Source: CAD feature listing. Evaluate the final solid. Frame: model axes, mm. Face numbers are marked on the shaded views. A direction names the side the tool comes from. Give positions to 0.01 mm unless a question says otherwise; leave off trailing zeros. Loops run counter-clockwise (first coordinate to the right, second up) from the corner with the lowest first, then second, coordinate; pieces in that order, holes last.
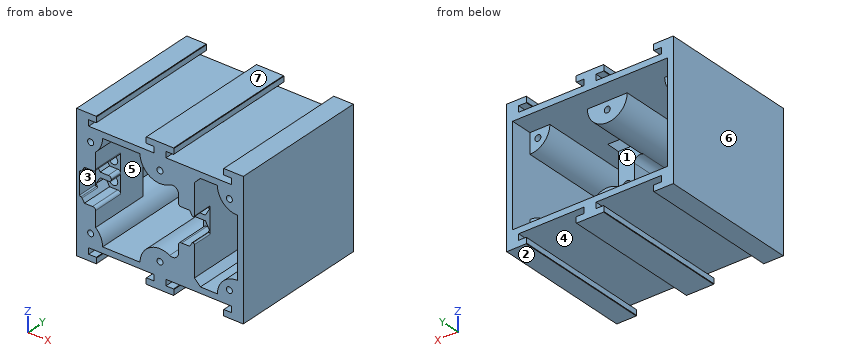
```python
from build123d import *

# Parameters (mm, degrees)
SKETCH1_R             = 1.5
BOSS_EXTRUDE6_DEPTH   = 59
BOSS_EXTRUDE6_2_DEPTH = 59
BOSS_EXTRUDE6_3_DEPTH = 59
BOSS_EXTRUDE6_4_DEPTH = 59
BOSS_EXTRUDE6_5_DEPTH = 59
BOSS_EXTRUDE6_6_DEPTH = 59
SKETCH2_W             = 83.65
SKETCH2_H             = 56
SKETCH2_W_2           = 77.65
SKETCH2_H_2           = 50
BOSS_EXTRUDE7_DEPTH   = 70
SKETCH3_R             = 2.1
SKETCH3_W             = 8
SKETCH3_H             = 50
BOSS_EXTRUDE8_DEPTH   = 30
CHAMFER1_SIZE         = 3
FILLET1_R             = 3
SKETCH4_R             = 2.1
CUT_EXTRUDE2_DEPTH    = 16
FILLET2_R             = 1.3
SKETCH5_W             = 8.8
SKETCH5_H             = 12
CUT_EXTRUDE3_DEPTH    = 10
FILLET3_R             = 0.6
SKETCH6_W             = 6
SKETCH6_H             = 6
BOSS_EXTRUDE9_DEPTH   = 70
CHAMFER3_SIZE         = 0.2


with BuildPart() as part:
    # Sketch1 → Boss-Extrude6 (new body)
    with BuildSketch(Plane(origin=(0, 0, 0), x_dir=(1, 0, 0), z_dir=(0, 1, 0))):
        with BuildLine():
            Line((-38.825, 15), (-38.825, 25))
            Line((-38.825, 25), (-28.825, 25))
            ThreePointArc((-28.825, 25), (-31.753932188, 17.928932188), (-38.825, 15))
        make_face()
        with Locations(Location((-34.825, 21, 0), (0, 0, 270))):
            Circle(SKETCH1_R, mode=Mode.SUBTRACT)
    extrude(amount=BOSS_EXTRUDE6_DEPTH)



with BuildPart() as body_2:
    # Sketch1 → Boss-Extrude6 2 (new body)
    with BuildSketch(Plane(origin=(0, 0, 0), x_dir=(1, 0, 0), z_dir=(0, 1, 0))):
        with BuildLine():
            Line((-38.825, -25), (-28.825, -25))
            ThreePointArc((-28.825, -25), (-31.753932188, -17.928932188), (-38.825, -15))
            Line((-38.825, -15), (-38.825, -25))
        make_face()
        with Locations(Location((-34.825, -21, 0), (0, 0, 270))):
            Circle(SKETCH1_R, mode=Mode.SUBTRACT)
    extrude(amount=BOSS_EXTRUDE6_2_DEPTH)


with BuildPart() as body_3:
    # Sketch1 → Boss-Extrude6 3 (new body)
    with BuildSketch(Plane(origin=(0, 0, 0), x_dir=(1, 0, 0), z_dir=(0, 1, 0))):
        with BuildLine():
            Line((38.825, -25), (38.825, -15))
            ThreePointArc((38.825, -15), (31.753932188, -17.928932188), (28.825, -25))
            Line((28.825, -25), (38.825, -25))
        make_face()
        with Locations(Location((34.825, -21, 0), (0, 0, 270))):
            Circle(SKETCH1_R, mode=Mode.SUBTRACT)
    extrude(amount=BOSS_EXTRUDE6_3_DEPTH)


with BuildPart() as body_4:
    # Sketch1 → Boss-Extrude6 4 (new body)
    with BuildSketch(Plane(origin=(0, 0, 0), x_dir=(1, 0, 0), z_dir=(0, 1, 0))):
        with BuildLine():
            Line((28.825, 25), (38.825, 25))
            Line((38.825, 25), (38.825, 15))
            ThreePointArc((38.825, 15), (31.753932188, 17.928932188), (28.825, 25))
        make_face()
        with Locations(Location((34.825, 21, 0), (0, 0, 270))):
            Circle(SKETCH1_R, mode=Mode.SUBTRACT)
    extrude(amount=BOSS_EXTRUDE6_4_DEPTH)


with BuildPart() as body_5:
    # Sketch1 → Boss-Extrude6 5 (new body)
    with BuildSketch(Plane(origin=(0, 0, 0), x_dir=(1, 0, 0), z_dir=(0, 1, 0))):
        with BuildLine():
            Line((10, -25), (-10, -25))
            ThreePointArc((-10, -25), (0, -15), (10, -25))
        make_face()
        with Locations(Location((0, -21, 0), (0, 0, 270))):
            Circle(SKETCH1_R, mode=Mode.SUBTRACT)
    extrude(amount=BOSS_EXTRUDE6_5_DEPTH)


with BuildPart() as body_6:
    # Sketch1 → Boss-Extrude6 6 (new body)
    with BuildSketch(Plane(origin=(0, 0, 0), x_dir=(1, 0, 0), z_dir=(0, 1, 0))):
        with BuildLine():
            Line((10, 25), (-10, 25))
            ThreePointArc((-10, 25), (0, 15), (10, 25))
        make_face()
        with Locations(Location((0, 21, 0), (0, 0, 270))):
            Circle(SKETCH1_R, mode=Mode.SUBTRACT)
    extrude(amount=BOSS_EXTRUDE6_6_DEPTH)


with BuildPart() as part_1:
    add(part.part)

    add(body_2.part)  # Boss-Extrude7 merges body 2

    add(body_3.part)  # Boss-Extrude7 merges body 3

    add(body_4.part)  # Boss-Extrude7 merges body 4

    add(body_5.part)  # Boss-Extrude7 merges body 5

    add(body_6.part)  # Boss-Extrude7 merges body 6
    # Sketch2 → Boss-Extrude7 (add)
    with BuildSketch(Plane(origin=(0, 0, 0), x_dir=(1, 0, 0), z_dir=(0, 1, 0))):
        Rectangle(SKETCH2_W, SKETCH2_H)
        Rectangle(SKETCH2_W_2, SKETCH2_H_2, mode=Mode.SUBTRACT)
    extrude(amount=BOSS_EXTRUDE7_DEPTH)

    # Sketch3 → Boss-Extrude8 (add)
    # profile 1 of 2: a face of its own
    with BuildSketch(Plane(origin=(0, 0, 0), x_dir=(1, 0, 0), z_dir=(0, 1, 0))):
        Polygon((-38.825, 0), (-38.825, 19), (-32.325, 19), (-32.325, -19), (-38.825, -19), align=None)
        with Locations(Location((-35.925, 4.8, 0), (0, 0, 270))):
            Circle(SKETCH3_R, mode=Mode.SUBTRACT)
        with Locations(Location((-35.925, -4.8, 0), (0, 0, 90))):
            Circle(SKETCH3_R, mode=Mode.SUBTRACT)
    # profile 2 of 2: a face of its own
    with BuildSketch(Plane(origin=(0, 0, 0), x_dir=(1, 0, 0), z_dir=(0, 1, 0))):
        with Locations((13.299000327, 0)):
            Rectangle(SKETCH3_W, SKETCH3_H)
        with Locations(Location((12.899000327, -4.8, 0), (0, 0, 270))):
            Circle(SKETCH3_R, mode=Mode.SUBTRACT)
        with Locations(Location((12.899000327, 4.8, 0), (0, 0, 90))):
            Circle(SKETCH3_R, mode=Mode.SUBTRACT)
    extrude(amount=BOSS_EXTRUDE8_DEPTH)

    # Chamfer1
    chamfer1_edges = [part_1.edges().sort_by_distance(p)[0] for p in [
        (13.649500163, 30, 25),
        (13.649500163, 30, -25),
        (17.299000327, 15, -25),
        (17.299000327, 15, 25),
    ]]
    chamfer(chamfer1_edges, length=CHAMFER1_SIZE)

    # Fillet1
    fillet1_edges = [part_1.edges().sort_by_distance(p)[0] for p in [
        (9.299000327, 15, -21.32187644),
        (9.299000327, 15, 21.32187644),
    ]]
    fillet(fillet1_edges, radius=FILLET1_R)

    # Sketch4 → Cut-Extrude2 (cut)
    # profile 1 of 4: a face of its own
    with BuildSketch(Plane.XZ):
        Polygon((-32.325, 4.035382907), (-32.325, 5.564617093), (-33.904274058, 8.3), (-37.945725942, 8.3), (-39.966451884, 4.8), (-37.945725942, 1.3), (-33.904274058, 1.3), align=None)
        with Locations(Location((-35.925, 4.8, 0), (0, 0, 270))):
            Circle(SKETCH4_R, mode=Mode.SUBTRACT)
    # profile 2 of 4: a face of its own
    with BuildSketch(Plane.XZ):
        Polygon((-32.325, -5.564617093), (-32.325, -4.035382907), (-33.904274058, -1.3), (-37.945725942, -1.3), (-39.966451884, -4.8), (-37.945725942, -8.3), (-33.904274058, -8.3), align=None)
        with Locations(Location((-35.925, -4.8, 0), (0, 0, 270))):
            Circle(SKETCH4_R, mode=Mode.SUBTRACT)
    # profile 3 of 4: a face of its own
    with BuildSketch(Plane.XZ):
        Polygon((10.878274385, -1.3), (9.299000327, -4.035382907), (9.299000327, -5.564617093), (10.878274385, -8.3), (14.919726269, -8.3), (16.940452211, -4.8), (14.919726269, -1.3), align=None)
        with Locations(Location((12.899000327, -4.8, 0), (0, 0, 270))):
            Circle(SKETCH4_R, mode=Mode.SUBTRACT)
    # profile 4 of 4: a face of its own
    with BuildSketch(Plane.XZ):
        Polygon((14.919726269, 1.3), (16.940452211, 4.8), (14.919726269, 8.3), (10.878274385, 8.3), (9.299000327, 5.564617093), (9.299000327, 4.035382907), (10.878274385, 1.3), align=None)
        with Locations(Location((12.899000327, 4.8, 0), (0, 0, 270))):
            Circle(SKETCH4_R, mode=Mode.SUBTRACT)
    extrude(amount=-CUT_EXTRUDE2_DEPTH, mode=Mode.SUBTRACT)

    # Fillet2
    # the kernel refuses this fillet: 1.3 mm, written as the material it takes off along each edge
    with BuildSketch(Plane(origin=(9.299000327, -10.012577226, -5.564617093), x_dir=(0.5000000000000003, 0, -0.8660254037844384), z_dir=(0, 1, 0)), Plane(origin=(9.299000327, -10.012577226, 4.035382907), x_dir=(0.5000000000000006, 0, -0.8660254037844383), z_dir=(0, 1, 0)), Plane(origin=(-32.325, -10.012577226, 5.564617093), x_dir=(-0.4999999999999981, 0, 0.8660254037844398), z_dir=(0, 1, 0)), Plane(origin=(-32.325, -10.012577226, -4.035382907), x_dir=(-0.5000000000000001, 0, 0.8660254037844386), z_dir=(0, 1, 0))) as fillet2_piece_1:
        with BuildLine():
            CenterArc((4.118458494, 0.87668242), FILLET2_R, 120, 102.405330947)
            Line((3.468458494, 2.002515445), (0, 0))
            Line((0, 0), (3.158548116, 0))
        make_face()
    extrude(amount=26.012577226, mode=Mode.SUBTRACT)
    with BuildSketch(Plane(origin=(9.299000327, -10.012577226, -4.035382907), x_dir=(0.4999999999999997, 0, 0.8660254037844388), z_dir=(0, 1, 0)), Plane(origin=(9.299000327, -10.012577226, 5.564617093), x_dir=(0.49999999999999944, 0, 0.866025403784439), z_dir=(0, 1, 0)), Plane(origin=(-32.325, -10.012577226, -5.564617093), x_dir=(-0.5000000000000004, 0, -0.8660254037844384), z_dir=(0, 1, 0)), Plane(origin=(-32.325, -10.012577226, 4.035382907), x_dir=(-0.5000000000000004, 0, -0.8660254037844383), z_dir=(0, 1, 0))) as fillet2_piece_2:
        with BuildLine():
            CenterArc((4.118458494, -0.87668242), FILLET2_R, 137.594669053, 102.405330947)
            Line((3.468458494, -2.002515445), (0, 0))
            Line((0, 0), (3.158548116, 0))
        make_face()
    extrude(amount=26.012577226, mode=Mode.SUBTRACT)

    # Sketch5 → Cut-Extrude3 (cut)
    with BuildSketch(Plane.XZ):
        with Locations((12.899000327, 0)):
            Rectangle(SKETCH5_W, SKETCH5_H)
        with Locations((-35.925, 0)):
            Rectangle(SKETCH5_W, SKETCH5_H)
    extrude(amount=-CUT_EXTRUDE3_DEPTH, mode=Mode.SUBTRACT)

    # Fillet3
    fillet3_edges = [part_1.edges().sort_by_distance(p)[0] for p in [
        (16.247631888, 5, 6),
        (16.247631888, 5, -6),
        (17.299000327, 5, -6),
        (17.299000327, 5, 6),
        (-39.273631561, 5, -6),
        (-39.273631561, 5, 6),
        (-40.325, 5, 6),
        (-40.325, 5, -6),
    ]]
    fillet(fillet3_edges, radius=FILLET3_R)

    # Sketch6 → Boss-Extrude9 (add)
    with BuildSketch(Plane(origin=(0, 0, 0), x_dir=(1, 0, 0), z_dir=(0, 1, 0))):
        Polygon((-7, 31), (-3, 31), (3, 31), (7, 31), (7, 34), (-7, 34), align=None)
        with Locations((0, 28)):
            Rectangle(SKETCH6_W, SKETCH6_H)
        with Locations((-38.825, 28)):
            Rectangle(SKETCH6_W, SKETCH6_H)
        Polygon((-41.825, 31), (-35.825, 31), (-31.825, 31), (-31.825, 34), (-41.825, 34), align=None)
        Polygon((41.825, 31), (41.825, 34), (31.825, 34), (31.825, 31), (35.825, 31), align=None)
        with Locations((38.825, 28)):
            Rectangle(SKETCH6_W, SKETCH6_H)
        with Locations((38.825, -28)):
            Rectangle(SKETCH6_W, SKETCH6_H)
        Polygon((41.825, -31), (35.825, -31), (31.825, -31), (31.825, -34), (41.825, -34), align=None)
        Polygon((-41.825, -31), (-41.825, -34), (-31.825, -34), (-31.825, -31), (-35.825, -31), align=None)
        with Locations((-38.825, -28)):
            Rectangle(SKETCH6_W, SKETCH6_H)
        Polygon((-7, -34), (7, -34), (7, -31), (3, -31), (-3, -31), (-7, -31), align=None)
        with Locations((0, -28)):
            Rectangle(SKETCH6_W, SKETCH6_H)
    extrude(amount=BOSS_EXTRUDE9_DEPTH)

    # Chamfer3
    chamfer3_edges = [part_1.edges().sort_by_distance(p)[0] for p in [
        (-31.825, 35, 31),
        (-31.825, 35, 34),
        (31.825, 35, 34),
        (31.825, 35, 31),
        (-31.825, 35, -34),
        (-31.825, 35, -31),
        (-7, 35, -31),
        (-7, 35, -34),
        (7, 35, -34),
        (7, 35, -31),
        (31.825, 35, -34),
        (31.825, 35, -31),
        (-7, 35, 34),
        (7, 35, 34),
        (-7, 35, 31),
        (7, 35, 31),
    ]]
    chamfer(chamfer3_edges, length=CHAMFER3_SIZE)


solid = part_1.part
```
(1) Section A-A, the plane x = 0. Return the cut outline in (y, z).
A:
outline: (0, -34) - (70, -34) - (70, -25) - (59, -25) - (59, -22.5) - (0, -22.5) - close; (0, -19.5) - (59, -19.5) - (59, -15) - (0, -15) - close; (0, 15) - (59, 15) - (59, 19.5) - (0, 19.5) - close; (0, 22.5) - (59, 22.5) - (59, 25) - (70, 25) - (70, 34) - (0, 34) - close
(2) Ray query, line 1 along X through (y, z) = (26.75, -4.8) (3 decimals); line 2 along X through (y, z) = (16, -30) (3 decimals); line 3 along X through (y, z) = (19, -14) (3 decimals). Return the intervals inside material, ascending.
A:
line 1: x = -41.825 to -38.025, -33.825 to -32.325, 9.299 to 10.799, 14.999 to 17.299, 38.825 to 41.825
line 2: x = -41.825 to -35.825, -3 to 3, 35.825 to 41.825
line 3: x = -41.825 to -32.325, 9.276 to 17.299, 38.825 to 41.825
(3) Section C-C, the plane y = 35. Count the separate pieces of the cut face and the enclosed holes in it, then the cut area to 3 significant figures.
A:
separate pieces: 1
enclosed holes: 7
area: 1,700 mm2
(4) Section B-B, the plane x = -19. Return the cut outline in (y, z), then the cut area to 3 significant figures.
A:
outline: (0, -28) - (70, -28) - (70, -25) - (0, -25) - close; (0, 25) - (70, 25) - (70, 28) - (0, 28) - close
area: 420 mm2
(5) Mould query, pull axis X, two halves, no side actions, for the marked faces 5, 6 and 7. Classes: pulls with the +X half, pulls with the -X half, needs draft (parallel to the pull), parting line crosses it, or undercut.
A:
face 5: undercut
face 6: pulls with the -X half
face 7: needs draft
(6) Reachability of the marked faces 1, 2, 3 and 4 from +Z, -Z, +X, -X, +Y, -Y: full face, straight path, thin tool, end or side. Return the list, or none.
A:
face 1: +Y
face 2: -Z, +X, -X, +Y, -Y
face 3: -Y
face 4: +Y, -Y
(7) First-contact query: pin 1 (4 mm diameter, centred on x = -14, y = 21.5, fed in from -Z); pin 2 (2.5 mm diameter, centred on x = 12.899, z = -4.8, fed in from +Y); pin 3 (4 mm diameter, centred on x = 23.5, y = 23, fed in from +Z); pin 4 (6 mm diameter, centred on x = 13, z = -5.5, fed in from +Y). Flat tips, straight axial feed; report the tip coordinate or a pass-through.
A:
pin 1: stops at z = -28
pin 2: passes through
pin 3: stops at z = 28
pin 4: stops at y = 30
